Here's how the part is built. I have some questions about the finished solid (model axes, mm). Coordinates: 2 decimals unless noted, no trailing zeros. Loops run counter-clockwise (first coordinate to the right, second up) from the corner with the lowest first, then second, coordinate; pieces in that order, holes last. Notation, with made-up numbers: (10.5, 20.5) - (33.5, 20.5) arc R6 cw to (33.5, 28.5) - close; hole circle Ø6 at (-37, -28.75). An arc over 180 degrees is marked (long way). Use a Markdown table: item, result.
```python
from build123d import *

# Parameters (mm, degrees)
SKETCH1_R      = 32.122013297
SKETCH1_R_2    = 24.775693006
EXTRUDE1_DEPTH = 10
FILLET1_R      = 2


with BuildPart() as part:
    # Sketch1 → Extrude1 (new body)
    with BuildSketch(Plane(origin=(0, 0, 0), x_dir=(1, 0, 0), z_dir=(0, 1, 0))):
        Circle(SKETCH1_R)
        Circle(SKETCH1_R_2, mode=Mode.SUBTRACT)
    extrude(amount=EXTRUDE1_DEPTH)

    # Fillet1
    fillet1_edges = [part.edges().sort_by_distance(p)[0] for p in [
        (-32.122013297, 0, 0),
        (-32.122013297, 10, 0),
        (-24.775693006, 0, 0),
        (-24.775693006, 10, 0),
    ]]
    fillet(fillet1_edges, radius=FILLET1_R)


solid = part.part
```
Q1. I want a section at D-D, the plane y = 1.25. Write out the boundary of the cut face in (x, z), then the cut area to 3 significant figures.
Check values:
| item | result |
|---|---|
| outline | circle Ø63.95 at (0, 0); hole circle Ø49.84 at (0, 0) |
| area | 1,260 mm^2 |
Q2. I want a section at B-B, the plane x = 0. Write out the boundary of the cut face in (y, z).
Check values:
| item | result |
|---|---|
| outline | (0, -30.12) arc R2 ccw to (2, -32.12) - (8, -32.12) arc R2 ccw to (10, -30.12) - (10, -26.78) arc R2 ccw to (8, -24.78) - (2, -24.78) arc R2 ccw to (0, -26.78) - close; (0, 26.78) arc R2 ccw to (2, 24.78) - (8, 24.78) arc R2 ccw to (10, 26.78) - (10, 30.12) arc R2 ccw to (8, 32.12) - (2, 32.12) arc R2 ccw to (0, 30.12) - close |
Q3. If we mould it in two halves opening along Z, with no side actions, what happens to faces 1 (the face through (11.43, 4.96, 21.98)), 2 (the face through (-27, 10, 2)), 3 (the face through (30.64, 4.96, -9.65))? For each: pulls with the +Z half, pulls with the -Z half, needs draft (parallel to the pull), parting line crosses it, or undercut.
Check values:
| item | result |
|---|---|
| face 1 | undercut |
| face 2 | needs draft |
| face 3 | parting line crosses it |
Q4. Will these pins go through, and if not, where does the flat tip stop? P1, Ø1.5, axis at x = 13, y = 8, coming from the +Z side; P2, Ø6, axis at x = 2, y = 2.5, coming from the +Z side; P3, Ø1, axis at x = -23.5, y = 8.5, coming from the +Z side.
Check values:
| item | result |
|---|---|
| P1 | z = 29.69 |
| P2 | z = 32.12 |
| P3 | z = 22.36 |
Q5. I want a section at A-A, the plane z = 0. Write out the boundary of the cut face in (x, y), then the cut area to 3 significant figures.
Check values:
| item | result |
|---|---|
| outline | (-32.12, 2) arc R2 ccw to (-30.12, 0) - (-26.78, 0) arc R2 ccw to (-24.78, 2) - (-24.78, 8) arc R2 ccw to (-26.78, 10) - (-30.12, 10) arc R2 ccw to (-32.12, 8) - close; (24.78, 2) arc R2 ccw to (26.78, 0) - (30.12, 0) arc R2 ccw to (32.12, 2) - (32.12, 8) arc R2 ccw to (30.12, 10) - (26.78, 10) arc R2 ccw to (24.78, 8) - close |
| area | 140 mm^2 |
Q6. Please list where these lines run through material, in increasing order: L1, parallel to Z at x = 0, y = 4.5; L2, parallel to X at y = 5.25, z = -13.5. Write a range as from..to.
Check values:
| item | result |
|---|---|
| L1 | -32.12..-24.78, 24.78..32.12 |
| L2 | -29.15..-20.77, 20.77..29.15 |
Q7. I want a section at C-C, the plane y = 7.25. Write out the boundary of the cut face in (x, z).
Check values:
| item | result |
|---|---|
| outline | circle Ø64.24 at (0, 0); hole circle Ø49.55 at (0, 0) |
